Geometry: final body of the model. Coordinates: model frame, mm. A direction names the side the tool comes from. Coordinates: 2 decimals unless noted, no trailing zeros. Write each loop counter-clockwise with the first axis right and the second up, starting at its lowest first coordinate (ties: lowest second). Pieces come first, ordered by that corner, then holes.
from build123d import *
from build123d.topology import SkipClean

# Parameters (mm, degrees)
SKETCH_1_W          = 9.5
SKETCH_1_H          = 9.5
EXTRUDE_2_DEPTH     = 5
FILLET_2_R          = 1
CUT_EXTRUDE_1_DEPTH = 34.132793262
EXTRUDE_3_DEPTH     = 5
EXTRUDE_5_DEPTH     = 2
EXTRUDE_6_DEPTH     = 2
EXTRUDE_7_DEPTH     = 2
EXTRUDE_8_DEPTH     = 2
EXTRUDE_START       = 2
EXTRUDE_10_DEPTH    = 2
SKETCH_15_R         = 3.5
EXTRUDE_11_DEPTH    = 58
SKETCH_16_W         = 9.8
SKETCH_16_H         = 9.8
EXTRUDE_12_DEPTH    = 10


with BuildPart() as part:
    # 草图1 → 凸台-拉伸2 (new body)
    with BuildSketch(Plane.XY):
        Polygon((-30.033755564, 13.067345411), (-14.533755564, 13.067345411), (-14.533755564, -2.432654589), (-30.033755564, -2.432654589), (-30.033755564, 10.067345411), align=None)
        with Locations((-22.283755564, 5.317345411)):
            Rectangle(SKETCH_1_W, SKETCH_1_H, mode=Mode.SUBTRACT)
    extrude(amount=EXTRUDE_2_DEPTH)

    # 圆角2
    fillet_2_edges = [part.edges().sort_by_distance(p)[0] for p in [
        (-30.033755564, 13.067345411, 2.5),
        (-14.533755564, 13.067345411, 2.5),
        (-14.533755564, -2.432654589, 2.5),
        (-30.033755564, -2.432654589, 2.5),
    ]]
    fillet(fillet_2_edges, radius=FILLET_2_R)

    # 草图2 → 切除-拉伸1 (cut, through all)
    with BuildSketch(Plane.XY.offset(5)):
        with BuildLine():
            ThreePointArc((-16.783755564, 5.317345411), (-16.974565419, 6.753486072), (-17.533755564, 8.089979537))
            Line((-17.533755564, 8.089979537), (-17.533755564, 2.544711284))
            ThreePointArc((-17.533755564, 2.544711284), (-16.974565419, 3.881204749), (-16.783755564, 5.317345411))
        make_face()
        with BuildLine():
            ThreePointArc((-19.511121437, 10.067345411), (-22.283755564, 10.817345411), (-25.056389691, 10.067345411))
            Line((-25.056389691, 10.067345411), (-22.283755564, 10.067345411))
            Line((-22.283755564, 10.067345411), (-19.511121437, 10.067345411))
        make_face()
        with BuildLine():
            Line((-27.033755564, 2.544711284), (-27.033755564, 8.089979537))
            ThreePointArc((-27.033755564, 8.089979537), (-27.783755564, 5.317345411), (-27.033755564, 2.544711284))
        make_face()
        with BuildLine():
            Line((-19.511121437, 0.567345411), (-22.283755564, 0.567345411))
            Line((-22.283755564, 0.567345411), (-25.056389691, 0.567345411))
            ThreePointArc((-25.056389691, 0.567345411), (-22.283755564, -0.182654589), (-19.511121437, 0.567345411))
        make_face()
    extrude(amount=-CUT_EXTRUDE_1_DEPTH, mode=Mode.SUBTRACT)

    # 草图4 → 凸台-拉伸3 (add)
    with SkipClean():  # the faces are left unmerged after this step: merging them gives an invalid solid
        with BuildSketch(Plane.XY.offset(5)):
            with BuildLine():
                Line((-25.056389691, 10.067345411), (-27.033755564, 10.067345411))
                Line((-27.033755564, 10.067345411), (-27.033755564, 8.089979537))
                ThreePointArc((-27.033755564, 8.089979537), (-26.17284286, 9.206432707), (-25.056389691, 10.067345411))
            make_face()
            with BuildLine():
                Line((-17.533755564, 10.067345411), (-19.511121437, 10.067345411))
                ThreePointArc((-19.511121437, 10.067345411), (-18.394668267, 9.206432707), (-17.533755564, 8.089979537))
                Line((-17.533755564, 8.089979537), (-17.533755564, 10.067345411))
            make_face()
            with BuildLine():
                Line((-17.533755564, 0.567345411), (-17.533755564, 2.544711284))
                ThreePointArc((-17.533755564, 2.544711284), (-18.394668267, 1.428258114), (-19.511121437, 0.567345411))
                Line((-19.511121437, 0.567345411), (-17.533755564, 0.567345411))
            make_face()
            with BuildLine():
                ThreePointArc((-25.056389691, 0.567345411), (-26.17284286, 1.428258114), (-27.033755564, 2.544711284))
                Line((-27.033755564, 2.544711284), (-27.033755564, 0.567345411))
                Line((-27.033755564, 0.567345411), (-25.056389691, 0.567345411))
            make_face()
        extrude(amount=-EXTRUDE_3_DEPTH)

    # 草图9 → 凸台-拉伸5 (add)
    with SkipClean():  # the faces are left unmerged after this step: merging them gives an invalid solid
        with BuildSketch(Plane.XZ.offset(2.432654589)):
            Polygon((-22.283755564, -5), (-22.283755564, 0), (-26.783755564, 0), (-23.283755564, -5), align=None)
            Polygon((-17.783755564, 0), (-22.283755564, 0), (-22.283755564, -5), (-21.283755564, -5), align=None)
        extrude(amount=-EXTRUDE_5_DEPTH)

    # 草图10 → 凸台-拉伸6 (add)
    with SkipClean():  # the faces are left unmerged after this step: merging them gives an invalid solid
        with BuildSketch(Plane(origin=(-14.533755564, 0, 0), x_dir=(0, 0, -1), z_dir=(1, 0, 0))):
            Polygon((5, 5.317345411), (0, 5.317345411), (0, 0.817345411), (5, 4.317345411), align=None)
            Polygon((0, 9.817345411), (0, 5.317345411), (5, 5.317345411), (5, 6.317345411), align=None)
        extrude(amount=-EXTRUDE_6_DEPTH)

    # 草图11 → 凸台-拉伸7 (add)
    with SkipClean():  # the faces are left unmerged after this step: merging them gives an invalid solid
        with BuildSketch(Plane.ZY.offset(30.033755564)):
            Polygon((0, 0.817345411), (0, 5.317345411), (-5, 5.317345411), (-5, 4.317345411), align=None)
            Polygon((-5, 5.317345411), (0, 5.317345411), (0, 9.817345411), (-5, 6.317345411), align=None)
        extrude(amount=-EXTRUDE_7_DEPTH)

    # 草图12 → 凸台-拉伸8 (add)
    with SkipClean():  # the faces are left unmerged after this step: merging them gives an invalid solid
        with BuildSketch(Plane(origin=(0, 13.067345411, 0), x_dir=(1, 0, 0), z_dir=(0, 1, 0))):
            Polygon((-26.783755564, 0), (-22.283755564, 0), (-22.283755564, 5), (-23.283755564, 5), align=None)
            Polygon((-22.283755564, 5), (-22.283755564, 0), (-17.783755564, 0), (-21.283755564, 5), align=None)
        extrude(amount=-EXTRUDE_8_DEPTH)

    # 草图13 → 凸台-拉伸10 (add)
    with SkipClean():  # the faces are left unmerged after this step: merging them gives an invalid solid
        with BuildSketch(Plane.XY.offset(5).offset(EXTRUDE_START)):
            with BuildLine():
                Line((-30.033755564, 12.067345411), (-30.033755564, -1.432654589))
                ThreePointArc((-30.033755564, -1.432654589), (-29.740862345, -2.13976137), (-29.033755564, -2.432654589))
                Line((-29.033755564, -2.432654589), (-15.533755564, -2.432654589))
                ThreePointArc((-15.533755564, -2.432654589), (-14.826648783, -2.13976137), (-14.533755564, -1.432654589))
                Line((-14.533755564, -1.432654589), (-14.533755564, 12.067345411))
                ThreePointArc((-14.533755564, 12.067345411), (-14.826648783, 12.774452192), (-15.533755564, 13.067345411))
                Line((-15.533755564, 13.067345411), (-29.033755564, 13.067345411))
                ThreePointArc((-29.033755564, 13.067345411), (-29.740862345, 12.774452192), (-30.033755564, 12.067345411))
            make_face()
        extrude(amount=-EXTRUDE_10_DEPTH)

    # 草图15 → 凸台-拉伸11 (add)
    with SkipClean():  # the faces are left unmerged after this step: merging them gives an invalid solid
        with BuildSketch(Plane.XY.offset(7)):
            with Locations(Location((-22.283755564, 5.317345411, 0), (0, 0, 180))):
                Circle(SKETCH_15_R)
        extrude(amount=EXTRUDE_11_DEPTH)

    # 草图16 → 凸台-拉伸12 (add)
    with SkipClean():  # the faces are left unmerged after this step: merging them gives an invalid solid
        with BuildSketch(Plane.XY.offset(65)):
            with Locations((-22.283755564, 5.317345411)):
                Rectangle(SKETCH_16_W, SKETCH_16_H)
        extrude(amount=EXTRUDE_12_DEPTH)


solid = part.part
Item 1: Pull-direction query (Z, two-part tool) for faces 1 (the flat face through (-23, 9, 65)), 2 (the flat face through (-22, 13.067, 2)), 3 (the flat face through (-22, -1, -5)), 4 (the flat face through (-26, 5, 7)); classes: released by +Z, released by -Z, zero draft, split by the parting line, or undercut.
Derived:
face 1: undercut
face 2: zero draft
face 3: released by -Z
face 4: undercut
Item 2: Section B-B, the plane z = 69.5. Output: boundary loops of the cut face in (x, y).
Derived:
outline: (-27.18, 0.42) - (-17.38, 0.42) - (-17.38, 10.22) - (-27.18, 10.22) - close
Item 3: Set-up query: faces 5 (the flat face through (-28.034, 5, -2)), 6 (the flat face through (-22, 11.067, -2)), 7 (the flat face through (-22, 0.417, 70)). Return all of +Z, -Z, +X, -X, +Y, -Y with unobstructed straight access to the full face (end or side cutting, diameter ignored); none if empty.
Derived:
face 5: -Z, +Y, -Y
face 6: -Z, +X, -X
face 7: +Z, +X, -X, -Y
Item 4: Section C-C, the plane z = 19.5. Output: boundary loops of the cut face in (x, y).
Derived:
outline: circle Ø7 at (-22.28, 5.32)
Item 5: Pin query (flat end, axial travel): pin 1 (8 mm diameter, centred on x = -25, z = 55.5, fed in from +Y); pin 2 (1 mm diameter, centred on x = -25.5, z = 43, fed in from +Y); pin 3 (5 mm diameter, centred on x = -21.5, y = 3.5, fed in from -Z). Return the tip coordinate at first contact, or that it passes through.
Derived:
pin 1: stops at y = 8.82
pin 2: stops at y = 7.52
pin 3: stops at z = 5
Item 6: Section A-A, the plane x = -22.5. Output: boundary loops of the cut face in (y, z).
Derived:
outline: (-2.43, -5) - (-0.43, -5) - (-0.43, 0) - (-0.18, 0) - (-0.18, 5) - (10.81, 5) - (10.81, 0) - (11.07, 0) - (11.07, -5) - (13.07, -5) - (13.07, 7) - (8.81, 7) - (8.81, 65) - (10.22, 65) - (10.22, 75) - (0.42, 75) - (0.42, 65) - (1.82, 65) - (1.82, 7) - (-2.43, 7) - close
Item 7: Material intervals for probe 1 along Z at (x, y) = (-18.75, 9.25); probe 2 along Z at (x, y) = (-24.25, 0.25); probe 3 along Z at (x, y) = (-23.5, 8), sorted ascending.
Derived:
probe 1: z = 5 to 7, 65 to 75
probe 2: z = 5 to 7
probe 3: z = 5 to 75
